Input: dimensioned drawing with shaded views. Units: mm. Origin: part minimum x, y, z. Round coordinates to 2 decimals unless told otherwise and drop trailing zeros. Loops run counter-clockwise (first coordinate to the right, second up) from the corner with the lowest first, then second, coordinate; pieces in that order, holes last.
1) Section D-D, the plane x = 3.5. Return loops of the section in (y, z).
2) Ray query, line 1 along Y through (x, z) = (2, 29); line 2 along Y through (x, z) = (21, 27); line 3 along Z through (x, y) = (26.5, 14.75). Return the intervals inside material, ascending.
3) Section C-C, the plane y = 6.5. State how many separate pieces and enclosed holes the cut face has, and give its area (3 significant figures).
4) Section B-B, the plane x = 25.5. Return loops of the section in (y, z), and give its area (3 significant figures).
5) First-contact query: pin 1 (6 mm diameter, centred on x = 24, y = 9, fed in from -Z) (1 decimal); pin 2 (2 mm diameter, centred on x = 9.5, y = 16, fed in from -Z); pin 3 (8.5 mm diameter, centred on y = 7, z = 11, fed in from -X); pin 4 (2 mm diameter, centred on y = 6.5, z = 29, fed in from -X). Flat tips, straight axial feed; report the tip coordinate or a pass-through.
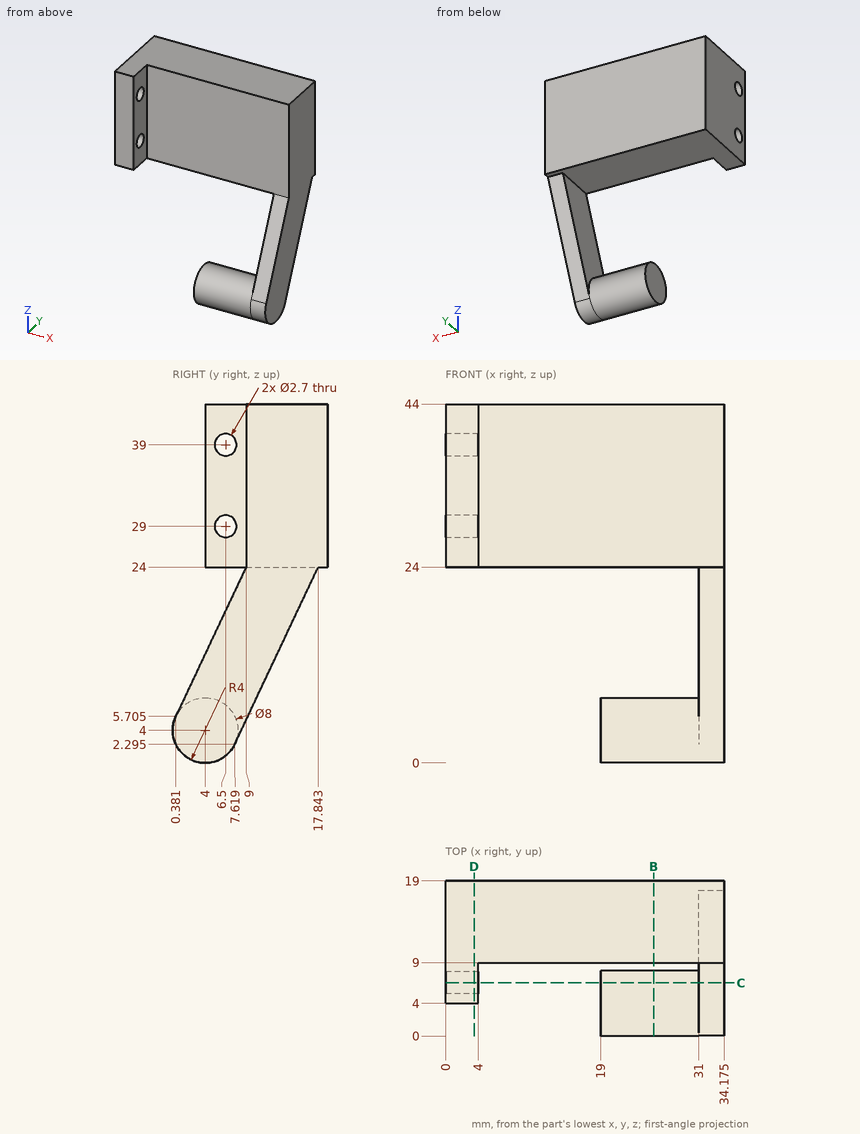
Final values:
1. outline: (4, 24) - (19, 24) - (19, 44) - (4, 44) - close; hole circle Ø2.7 at (6.5, 29); hole circle Ø2.7 at (6.5, 39)
2. line 1: y = 4 to 5.15, 7.85 to 19
2. line 2: y = 9 to 19
2. line 3: z = 24 to 44
3. separate pieces: 4
3. enclosed holes: 0
3. area: 190 mm2
4. outline: circle Ø8 at (4, 4); (9, 24) - (19, 24) - (19, 44) - (9, 44) - close
4. area: 250 mm2
5. pin 1: stops at z = 0.5
5. pin 2: stops at z = 24
5. pin 3: stops at x = 19
5. pin 4: passes through
